Geometry: final body of the model. Coordinates: model frame, mm. Face numbers are marked on the shaded views. A direction names the side the tool comes from. Give positions to 0.01 mm unless a question says otherwise; leave off trailing zeros. Write each loop counter-clockwise with the first axis right and the second up, starting at its lowest first coordinate (ties: lowest second). Pieces come first, ordered by that corner, then holes. Notation, with made-up numbers: (-27, -27.75) - (6, -27.75) arc R26 ccw to (6, 4.25) - close; hole circle Ø2 at (61, 5). An arc over 180 degrees is marked (long way). Return JSON: item names as keys, results as strings.
Autodesk Inventor part; units mm, degrees
ref_plane "Work Plane1" through (22.5, 0, 0) normal (1, 0, 0) x (0, 0, -1)
ref_plane "YZ Plane" through (0, 0, 0) normal (1, 0, 0) x (0, 1, 0)
ref_plane "XZ Plane" through (0, 0, 0) normal (0, 1, 0) x (-1, 0, 0)
sketch "Sketch1" plane through (0, 0, 0) normal (0, 1, 0) x (-1, 0, 0)
  line L0 (0, 0) -> (-45, 0)
  line L1 (-45, 0) -> (-45, -10)
  line L2 (-45, -10) -> (0, -10)
  line L3 (0, -10) -> (0, 0)
  dimension "d0" = 10
  dimension "d1" = 45
extrude "Extrusion1" add sketch "Sketch1" along normal blind 2.5
sketch "Sketch2" plane through (0, 0, 0) normal (0, -1, 0) x (1, 0, 0)
  line L0 (0, 0) -> (45, 0)
  line L1 (0, -10) -> (0, 0)
  line L2 (45, -10) -> (0, -10)
  line L3 (45, 0) -> (45, -10)
  line L4 (0, 0) -> (45, 0)
  line L5 (2.5, 0) -> (2.5, -10)
  line L6 (42.5, 0) -> (42.5, -10)
  line L7 (45, -10) -> (0, -10)
  dimension "d4" = 2.5
  dimension "d5" = 2.5
extrude "Extrusion2" add sketch "Sketch2" along normal blind 3 contours L0 L5 L2 L1 | L0 L3 L2 L6
sketch "Sketch3" plane through (0, -3, 0) normal (0, -1, 0) x (1, 0, 0)
  line L0 (0, -10) -> (2.5, -10)
  line L1 (2.5, -10) -> (2.5, 0)
  line L2 (2.5, 0) -> (0, 0)
  line L3 (0, 0) -> (0, -10)
  line L4 (0, 0) -> (-7, 0)
  line L5 (-7, 0) -> (-7, -10)
  line L6 (-7, -10) -> (0, -10)
  line L7 (0, -10) -> (0, 0)
  line L8 (0, -10) -> (2.5, -10)
  dimension "d8" = 7
extrude "Extrusion3" add sketch "Sketch3" against normal blind 2.5 contours L6 L5 L4 L3
sketch "Sketch4" plane through (0, -0.5, 0) normal (0, 1, 0) x (1, 0, 0)
  line L0 (-7, 0) -> (0, 0)
  line L1 (0, 10) -> (0, 0)
  line L2 (0, 10) -> (-7, 10)
  line L3 (-7, 10) -> (-7, 0)
  line L4 (0, 10) -> (0, 0) construction
  line L5 (0, 5) -> (-3, 5) construction
  circle A0 centre (-3, 5) radius 1.6
  dimension "d11" = 3
  dimension "d12" = 3.2
extrude "Extrusion4" cut sketch "Sketch4" against normal up to surface (2.5 mm away) contours A0
ref_plane "Work Plane1" through (22.5, 0, 0) normal (1, 0, 0) x (0, 0, -1)
fillet "Fillet1" radius 4 2 edges at (-7, -1.75, 0) (-7, -1.75, -10)
mirror "Mirror1" about plane through (22.5, 0, 0) normal (1, 0, 0) of "Fillet1", "Extrusion4", "Extrusion3"
fillet "Fillet3" radius 2 4 edges at (2.5, 0, -5) (42.5, 0, -5) (0, 2.5, -5) (45, 2.5, -5)
equation "\"d2\" = wall_thickness"
equation "\"d4\" = wall_thickness"
equation "\"d5\" = wall_thickness"
equation "\"d9\" = wall_thickness"
equation "\"d13\" = wall_thickness"
equation "\"wall_thickness\" = 2.5"
properties part number "battery_mount_1s_500mah"
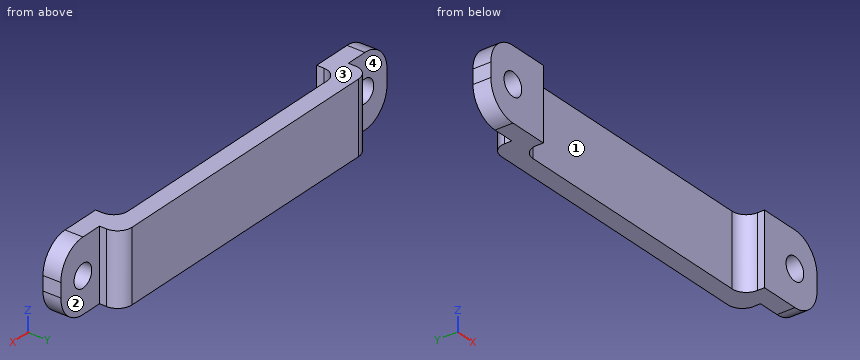
Q1. Section query B-B, the plane z = -8.75. Return the cut outline in (x, y), plus the area to 3 significant figures.
Answer key:
{"outline": "(-5.9, -3) - (2.5, -3) - (2.5, -2) arc R2 cw to (4.5, 0) - (40.5, 0) arc R2 cw to (42.5, -2) - (42.5, -3) - (50.9, -3) - (50.9, -0.5) - (45, -0.5) - (45, 0.5) arc R2 ccw to (43, 2.5) - (2, 2.5) arc R2 ccw to (0, 0.5) - (0, -0.5) - (-5.9, -0.5) - close", "area": "157 mm^2"}
Q2. Pin query (flat end, axial travel): P1, Ø1.5, axis at x = 3.5, z = -2, coming from the -Y side; P2, Ø1.5, axis at y = 1.5, z = -4, coming from the +X side; P3, Ø1, axis at y = 2, z = -5, coming from the -X side. Return the tip coordinate at first contact, or that it passes through.
Answer key:
{"P1": "stops at y = -1.03", "P2": "stops at x = 44.98", "P3": "stops at x = 0.27"}
Q3. Section query D-D, the plane y = 1.9. Return the cut outline in (x, z).
Answer key:
{"outline": "(0.57, -10) - (44.43, -10) - (44.43, 0) - (0.57, 0) - close"}
Q4. Set-up query: the marked faces 1, 2, 3 and 4. Return all of +Z, -Z, +X, -X, +Y, -Y with unobstructed straight access to the full face (end or side cutting, diameter ignored); none if empty.
Answer key:
{"face 1": "+Z, -Z, -Y", "face 2": "+Z, -Z, +X, +Y", "face 3": "+Z, +X, -X, +Y, -Y", "face 4": "+Z, -Z, -X, +Y"}
Q5. Section query C-C, the plane x = 13. Return the cut outline in (y, z).
Answer key:
{"outline": "(0, -10) - (2.5, -10) - (2.5, 0) - (0, 0) - close"}
Q6. Material intervals for probe 1 along X at (y, z) = (-2.3, -5); probe 2 along Z at (x, y) = (-3, -1.3); probe 3 along X at (y, z) = (-1.55, -5), sorted ascending. Write a range as [from, to].
Answer key:
{"probe 1": "x = [-7, -4.6], [-1.4, 2.5], [42.5, 46.4], [49.6, 52]", "probe 2": "z = [-10, -6.6], [-3.4, 0]", "probe 3": "x = [-7, -4.6], [-1.4, 2.55], [42.45, 46.4], [49.6, 52]"}
Q7. Section query A-A, the plane z = -5. Return the cut outline in (x, y).
Answer key:
{"outline": "(-7, -3) - (-4.6, -3) - (-4.6, -0.5) - (-7, -0.5) - close; (-1.4, -3) - (2.5, -3) - (2.5, -2) arc R2 cw to (4.5, 0) - (40.5, 0) arc R2 cw to (42.5, -2) - (42.5, -3) - (46.4, -3) - (46.4, -0.5) - (45, -0.5) - (45, 0.5) arc R2 ccw to (43, 2.5) - (2, 2.5) arc R2 ccw to (0, 0.5) - (0, -0.5) - (-1.4, -0.5) - close; (49.6, -3) - (52, -3) - (52, -0.5) - (49.6, -0.5) - close"}
